Source: CAD feature listing. Evaluate the final solid. Frame: model axes, mm. A direction names the side the tool comes from. Round coordinates to 2 decimals unless told otherwise and drop trailing zeros. Write each loop counter-clockwise with the first axis right and the second up, starting at its lowest first coordinate (ties: lowest second). Pieces come first, ordered by that corner, then holes. Notation, with made-up numbers: M 61.25,-38.75 L 111.25,-38.75 A26 cw 111.25,-10.75 Z; hole C 59.25,-13 d2. An arc over 180 degrees is marked long. Answer in a Markdown table with one row per item.
Autodesk Inventor part; units mm, degrees
ref_plane "Work Plane1" through (0, -2, 0) normal (0, -1, 0) x (1, 0, 0)
ref_plane "YZ Plane" through (0, 0, 0) normal (1, 0, 0) x (0, 1, 0)
ref_plane "XZ Plane" through (0, 0, 0) normal (0, 1, 0) x (-1, 0, 0)
sketch "Sketch1" plane through (0, 0, 0) normal (0, 1, 0) x (-1, 0, 0)
  circle A0 centre (0, 0) radius 19
  circle A1 centre (0, 0) radius 16
  dimension "d0" = 38
  dimension "d1" = 3
extrude "Extrusion1" add sketch "Sketch1" along normal blind 25
sketch "Sketch2" plane through (0, 0, 0) normal (0, -1, 0) x (1, 0, 0)
  circle A0 centre (0, 0) radius 22
  circle A1 centre (0, 0) radius 19
  dimension "d4" = 3
extrude "Extrusion2" add sketch "Sketch2" along normal blind 2 contours A0 | A1
ref_plane "Work Plane1" through (0, -2, 0) normal (0, -1, 0) x (1, 0, 0)
sketch "Sketch3" plane through (0, -2, 0) normal (0, -1, 0) x (1, 0, 0)
  circle A0 centre (0, 0) radius 2.125
  line L0 (1.625, -4.5) -> (1.625, 4.5)
  point P0 (1.625, -1.3693)
  point P1 (1.625, 1.3693)
  dimension "d8" = 4.25
  dimension "d9" = 9
  dimension "d10" = 4.5
  dimension "d11" = 1.625
extrude "Extrusion3" cut sketch "Sketch3" against normal blind 28 contours L0 A0 picked at (0.375, 0)
sketch "Sketch4" plane through (0, 0, 0) normal (0, 1, 0) x (1, 0, 0)
  circle A0 centre (0, 0) radius 5
  circle A1 centre (0, 0) radius 2
  line L0 (1.5, -1.3229) -> (1.5, 1.3229)
  line L1 (1.5, 1.3229) -> (1.5, -1.3229)
  dimension "d14" = 3
  dimension "d15" = 4
extrude "Extrusion4" add sketch "Sketch4" along normal blind 6 contours A0 | A1 L0 picked at (1.5908, -0.3089)
chamfer "Chamfer1" distance 1 angle 45 1 edges at (-22, -2, 0)
chamfer "Chamfer2" distance 1 angle 45 2 edges at (16, 0, 0) (-5, 0, 0)
properties part number "Kolo" material "Glass"
Q1. Section D-D (y = 22.5). Return loops of the section in (x, z), and give its area (3 significant figures).
Solutions:
| item | result |
|---|---|
| outline | C 0,0 d38; hole C 0,0 d32 |
| area | 330 mm2 |
Q2. Material intervals for probe 1 along Y at (x, z) = (-4, -19); probe 2 along X at (y, z) = (23, -6); probe 3 along X at (y, z) = (7.25, -2), sorted ascending.
Solutions:
| item | result |
|---|---|
| probe 1 | y = -2 to 0 |
| probe 2 | x = -18.03 to -14.83, 14.83 to 18.03 |
| probe 3 | x = -18.89 to -15.87, 15.87 to 18.89 |
Q3. Pull-direction query (Z, two-part tool) for faces 1 (the flat face through (1.625, -1, 0)), 2 (the cylindrical face through (-8.767, 12.325, 16.856)), 3 (the flat face through (-7, 0, 18)); classes: pulls with the +Z half, pulls with the -Z half, needs draft (parallel to the pull), parting line crosses it, or undercut.
Solutions:
| item | result |
|---|---|
| face 1 | undercut |
| face 2 | parting line crosses it |
| face 3 | needs draft |
Q4. Access query for faces 4 (the flat face through (4, -2, 0)), 5 (the flat face through (1.5, 3, 0)), 6 (the cylindrical face through (-2.124, -1.014, 0.073)), 7 (the cylindrical face through (3.47, 12.83, 15.62)). Directions: +Z, -Z, +X, -X, +Y, -Y. A direction counts if a zero-diameter tool reaches every point of the face in a straight line with its end or side. Return the directions, or none.
Solutions:
| item | result |
|---|---|
| face 4 | +Z, -Z, +X, -X, -Y |
| face 5 | +Y, -Y |
| face 6 | -Y |
| face 7 | +Y |
Q5. Section C-C (y = 3). Return loops of the section in (x, z).
Solutions:
| item | result |
|---|---|
| outline | C 0,0 d38; C 0,0 d10; hole C 0,0 d32; hole M 1.5,-1.32 L 1.5,1.32 A2 ccw long Z |
Q6. Contact query for flat-ended pins moving along their axis: pin 1 Ø11 at (x, z) = (1, -1.5) entering from +Y; pin 2 Ø6 at (y, z) = (19, 11.5) entering from -X; pin 3 Ø1.5 at (x, y) = (-12, 12) entering from -Z; pin 4 Ø4.5 at (x, z) = (0, 0) entering from -Y. Output: stop coordinate, or through.
Solutions:
| item | result |
|---|---|
| pin 1 | stops at y = 6 |
| pin 2 | stops at x = -16.99 |
| pin 3 | stops at z = -15.31 |
| pin 4 | stops at y = -2 |
